Here's how the part is built. I have some questions about the finished solid (model axes, mm). Face numbers are marked on the shaded views. A direction names the side the tool comes from. Give positions to 0.01 mm unless a question says otherwise; leave off trailing zeros. Write each loop counter-clockwise with the first axis right and the second up, starting at its lowest first coordinate (ties: lowest second). Pieces come first, ordered by that corner, then holes. Notation, with made-up numbers: M 67.25,70 L 90.25,70 A16 cw 90.25,85 Z; hole C 68,52.5 d5. An arc over 180 degrees is marked long. Use one line per item in the form item = value. Start each with the question number.
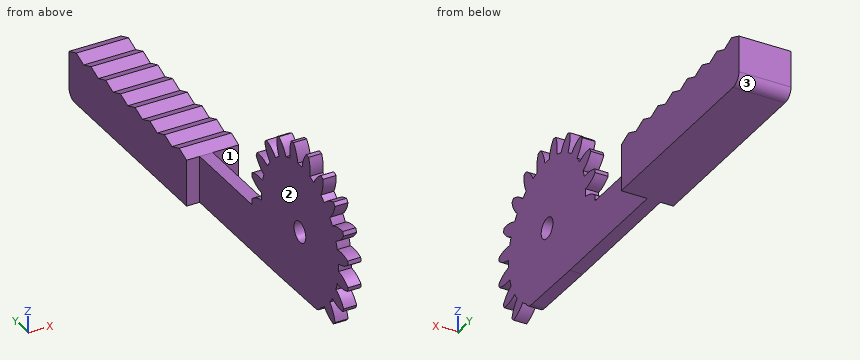
from build123d import *

# Parameters (mm, degrees)
BASPROSKE_W         = 2.5
BASPROSKE_H         = 16.5
TOOTHCUT_DEPTH      = 24.468063405
TEETHCUTS_COUNT     = 20
TEETHCUTS_ANGLE     = 342
BORSKE_R            = 2
BORE_DEPTH          = 50.0000508
SKETCH1_W           = 9
SKETCH1_H           = 70
BOSS_EXTRUDE2_DEPTH = 2.5
BOSS_EXTRUDE3_DEPTH = 2.5
LPATTERN2_COUNT     = 8
LPATTERN2_PITCH     = 5
CUT_EXTRUDE1_DEPTH  = 3
FILLET3_R           = 2
FILLET4_R           = 2
BOSS_EXTRUDE4_START = -2.5
BOSS_EXTRUDE4_DEPTH = 2.5
BOSS_EXTRUDE5_DEPTH = 5


with BuildPart() as part:
    # BasProSke → Base-Revolve (revolve)
    with BuildSketch(Plane(origin=(0, 0, 0), x_dir=(1, 0, 0), z_dir=(0, 1, 0)), mode=Mode.PRIVATE) as base_revolve_sk:
        with Locations((1.25, 8.25)):
            Rectangle(BASPROSKE_W, BASPROSKE_H)
    revolve(base_revolve_sk.sketch.rotate(Axis((-10, 0, 0), (1, 0, 0)), 180), axis=Axis((-10, 0, 0), (1, 0, 0)))

    # TooCutSke → ToothCut (cut, through all)
    with BuildSketch(Plane(origin=(0, 0, 0), x_dir=(0, 0, -1), z_dir=(1, 0, 0))):
        with BuildLine():
            ThreePointArc((0.74381438, 13.102904875), (0, 13.124), (-0.74381438, 13.102904875))
            ThreePointArc((-0.74381438, 13.102904875), (-1.226473103, 14.852072512), (-2.209965745, 16.376962373))
            ThreePointArc((-2.209965745, 16.376962373), (0, 16.5254), (2.209965745, 16.376962373))
            ThreePointArc((2.209965745, 16.376962373), (1.226473103, 14.852072512), (0.74381438, 13.102904875))
        make_face()
    toothcut = extrude(amount=TOOTHCUT_DEPTH, mode=Mode.SUBTRACT)

    # TeethCuts: ToothCut ×20 about axis
    teethcuts_axis = Axis((-10, 0, 0), (1, 0, 0))
    for i in range(1, TEETHCUTS_COUNT):
        add(toothcut.rotate(teethcuts_axis, i * TEETHCUTS_ANGLE / (TEETHCUTS_COUNT - 1)), mode=Mode.SUBTRACT)

    # BorSke → Bore (cut, symmetric)
    with BuildSketch(Plane(origin=(0, 0, 0), x_dir=(0, 0, -1), z_dir=(1, 0, 0))):
        with Locations(Location((0, 0, 0), (0, 0, 180))):
            Circle(BORSKE_R)
    extrude(amount=BORE_DEPTH, both=True, mode=Mode.SUBTRACT)

    # Sketch1 → Boss-Extrude2 (add)
    with BuildSketch(Plane(origin=(2.5, 0, 0), x_dir=(0, 0, -1), z_dir=(1, 0, 0))):
        with Locations((7.841610769, 39.08106639)):
            Rectangle(SKETCH1_W, SKETCH1_H)
    extrude(amount=-BOSS_EXTRUDE2_DEPTH)

    # Sketch2 → Boss-Extrude3 (add)
    with BuildSketch(Plane(origin=(2.5, 0, 0), x_dir=(0, 0, -1), z_dir=(1, 0, 0))):
        Polygon((2.341610769, 71.58106639), (3.341610769, 69.08106639), (3.341610769, 74.08106639), align=None)
    boss_extrude3 = extrude(amount=-BOSS_EXTRUDE3_DEPTH)

    # LPattern2: Boss-Extrude3 ×8
    with Locations(*[(0, -i * LPATTERN2_PITCH, 0) for i in range(1, LPATTERN2_COUNT)]):
        add(boss_extrude3)

    # Sketch3 → Cut-Extrude1 (cut)
    with BuildSketch(Plane(origin=(2.5, 0, 0), x_dir=(0, 0, -1), z_dir=(1, 0, 0))):
        Polygon((12.341610769, 7.640465379), (11.943579641, -16.474016898), (28.120591599, -19.002507116), (23.794346737, 10.948418847), align=None)
    extrude(amount=-CUT_EXTRUDE1_DEPTH, mode=Mode.SUBTRACT)

    # Fillet3
    # the kernel refuses this fillet: 2 mm, written as the material it takes off along each edge
    with BuildSketch(Plane(origin=(8.029722145, -7.563673717, -12.090652836), x_dir=(0, 0.40305029289493355, 0.9151778304773931), z_dir=(-1, 0, 0))) as fillet3_piece_1:
        with BuildLine():
            CenterArc((2.701383145, 1.26292574), FILLET3_R, 157.176626249, 61.981506818)
            Line((0.857973168, 2.038708994), (0.821104969, 2.054224659))
            Line((0.821104969, 2.054224659), (-0.0368682, 0.015515665))
            Line((-0.0368682, 0.015515665), (-0.003835236, -0.039815713))
            ThreePointArc((-0.003835236, -0.039815713), (0.575285457, -0.067643125), (1.119554669, -0.025258515))
            Line((1.119554669, -0.025258515), (1.150570914, 0))
        make_face()
    extrude(amount=13.55944429, mode=Mode.SUBTRACT)

    # Fillet4
    fillet4_edges = [part.edges().sort_by_distance(p)[0] for p in [
        (1.25, 74.08106639, -12.341610769),
    ]]
    fillet(fillet4_edges, radius=FILLET4_R)

    # Sketch5 → Boss-Extrude4 (add)
    with BuildSketch(Plane(origin=(2.5, 0, 0), x_dir=(0, 0, -1), z_dir=(1, 0, 0)).offset(BOSS_EXTRUDE4_START)):
        with BuildLine():
            ThreePointArc((3.341610769, 15.036857875), (3.187495997, 15.643253498), (2.971070911, 16.230303067))
            Line((2.971070911, 16.230303067), (3.341610769, 16.389315184))
            Line((3.341610769, 16.389315184), (3.341610769, 15.036857875))
        make_face()
    extrude(amount=BOSS_EXTRUDE4_DEPTH)

    # Sketch6 → Boss-Extrude5 (add, symmetric)
    with BuildSketch(Plane(origin=(2.5, 0, 0), x_dir=(0, 0, -1), z_dir=(1, 0, 0))):
        with BuildLine():
            Line((3.341610769, 34.08106639), (12.341610769, 34.08106639))
            Line((12.341610769, 34.08106639), (12.341610769, 72.08106639))
            ThreePointArc((12.341610769, 72.08106639), (11.755824331, 73.495279952), (10.341610769, 74.08106639))
            Line((10.341610769, 74.08106639), (3.341610769, 74.08106639))
            Line((3.341610769, 74.08106639), (2.341610769, 71.58106639))
            Line((2.341610769, 71.58106639), (3.341610769, 69.08106639))
            Line((3.341610769, 69.08106639), (2.341610769, 66.58106639))
            Line((2.341610769, 66.58106639), (3.341610769, 64.08106639))
            Line((3.341610769, 64.08106639), (2.341610769, 61.58106639))
            Line((2.341610769, 61.58106639), (3.341610769, 59.08106639))
            Line((3.341610769, 59.08106639), (2.341610769, 56.58106639))
            Line((2.341610769, 56.58106639), (3.341610769, 54.08106639))
            Line((3.341610769, 54.08106639), (2.341610769, 51.58106639))
            Line((2.341610769, 51.58106639), (3.341610769, 49.08106639))
            Line((3.341610769, 49.08106639), (2.341610769, 46.58106639))
            Line((2.341610769, 46.58106639), (3.341610769, 44.08106639))
            Line((3.341610769, 44.08106639), (2.341610769, 41.58106639))
            Line((2.341610769, 41.58106639), (3.341610769, 39.08106639))
            Line((3.341610769, 39.08106639), (2.341610769, 36.58106639))
            Line((2.341610769, 36.58106639), (3.341610769, 34.08106639))
        make_face()
    extrude(amount=BOSS_EXTRUDE5_DEPTH, both=True)


solid = part.part
1) Will these pins go through, and if not, where does the flat tip stop? P1, Ø0.8, axis at x = -1, z = -7.5, coming from the -Y side; P2, Ø1.5, axis at y = 4, z = 2, coming from the -X side; P3, Ø3, axis at y = -3, z = 6.5, coming from the +X side.
2) On a 3-axis mill with a long thin cutter (end or side, diameter ignored), from which of +Z, -Z, +X, -X, +Y, -Y can I reach the whole of each face in a straight line? I mean the marked faces 1, 2 and 3. Say none if no direction works.
3) Suppose I cut it at B-B, the plane z = -6. List the corners of the cut face in (x, y) for me.
4) Suppose I cut it at C-C, the plane y = 30. List the corners of the cut face in (x, z) for me.
5) Please list where these lines run through material, in increasing order: line 1 (Y direction, x = 0.8, z = 0); line 2 (X direction, y = 19.5, z = -7.25); line 3 (Y direction, x = 1, z = 10.25).
6) Suppose I cut it at A-A, the plane x = 6.5. List the corners of the cut face in (y, z) for me, and give its area (3 significant figures).
Checks:
q1.P1 = 34.08
q1.P2 = 0
q1.P3 = 2.5
q2.face_1 = +Z, -Z, +X, -Y
q2.face_2 = +Z, -Z, -X, -Y
q2.face_3 = -Z, +X, -X, +Y
q3.outline = M -2.5,34.08 L 0,34.08 L 0,-14 L 2.5,-14 L 2.5,34.08 L 7.5,34.08 L 7.5,74.08 L -2.5,74.08 Z
q4.outline = M 0,-12.34 L 2.5,-12.34 L 2.5,-3.34 L 0,-3.34 Z
q5.line_1 = -13.12 to -2, 2 to 13.12
q5.line_2 = 0 to 2.5
q5.line_3 = -11.56 to -8.39, -8.2 to 8.2, 8.39 to 11.56
q6.outline = M 34.08,-12.34 L 72.08,-12.34 A2 ccw 74.08,-10.34 L 74.08,-3.34 L 71.58,-2.34 L 69.08,-3.34 L 66.58,-2.34 L 64.08,-3.34 L 61.58,-2.34 L 59.08,-3.34 L 56.58,-2.34 L 54.08,-3.34 L 51.58,-2.34 L 49.08,-3.34 L 46.58,-2.34 L 44.08,-3.34 L 41.58,-2.34 L 39.08,-3.34 L 36.58,-2.34 L 34.08,-3.34 Z
q6.area = 379 mm^2
